Geometry: final body of the model. Coordinates: model frame, mm. A direction names the side the tool comes from. Give positions to 0.01 mm unless a question says otherwise; leave off trailing zeros. Loops run counter-clockwise (first coordinate to the right, second up) from the corner with the lowest first, then second, coordinate; pieces in that order, holes last. Notation, with made-up numbers: (73.25, 82.25) - (108.25, 82.25) arc R24 cw to (108.25, 106.25) - close; hole circle Ø5 at (-22.5, -37.75). An arc over 180 degrees is marked (long way). Answer in a Markdown table with one row per item.
from build123d import *

# Parameters (mm, degrees)
BOSS_EXTRUDE1_DEPTH = 36
SKETCH3_R           = 8.75
SKETCH3_R_2         = 8
CUT_EXTRUDE1_DEPTH  = 10
CUT_EXTRUDE2_DEPTH  = 2
SKETCH5_R           = 2.5
CUT_EXTRUDE3_DEPTH  = 1
SKETCH6_R           = 0.5
CUT_EXTRUDE4_DEPTH  = 5


with BuildPart() as part:
    # Sketch1 → Boss-Extrude1 (new body)
    with BuildSketch(Plane.XY):
        with BuildLine():
            Line((-77.5, 12.5), (77.5, 12.5))
            ThreePointArc((77.5, 12.5), (90, 0), (77.5, -12.5))
            Line((77.5, -12.5), (-77.5, -12.5))
            ThreePointArc((-77.5, -12.5), (-90, 0), (-77.5, 12.5))
        make_face()
    extrude(amount=-BOSS_EXTRUDE1_DEPTH)

    # Sketch3 → Cut-Extrude1 (cut)
    with BuildSketch(Plane.XY):
        with Locations((-28.5, 0)):
            Circle(SKETCH3_R)
        with Locations((18.5, 0)):
            Circle(SKETCH3_R_2)
        with Locations((44.5, 0)):
            Circle(SKETCH3_R_2)
    extrude(amount=-CUT_EXTRUDE1_DEPTH, mode=Mode.SUBTRACT)

    # Sketch4 → Cut-Extrude2 (cut)
    with BuildSketch(Plane.XY):
        with BuildLine():
            Line((-47.25, 9.5), (-20.75, 9.5))
            ThreePointArc((-20.75, 9.5), (-11.25, 0), (-20.75, -9.5))
            Line((-20.75, -9.5), (-47.25, -9.5))
            ThreePointArc((-47.25, -9.5), (-56.75, 0), (-47.25, 9.5))
        make_face()
        with BuildLine():
            Line((18, 9.5), (45, 9.5))
            ThreePointArc((45, 9.5), (54.5, 0), (45, -9.5))
            Line((45, -9.5), (18, -9.5))
            ThreePointArc((18, -9.5), (8.5, 0), (18, 9.5))
        make_face()
    extrude(amount=-CUT_EXTRUDE2_DEPTH, mode=Mode.SUBTRACT)

    # Sketch5 → Cut-Extrude3 (cut)
    with BuildSketch(Plane.XY):
        with Locations((72.5, -5.85958214)):
            Circle(SKETCH5_R)
        with Locations((-72.5, -5.85958214)):
            Circle(SKETCH5_R)
    extrude(amount=-CUT_EXTRUDE3_DEPTH, mode=Mode.SUBTRACT)

    # Sketch6 → Cut-Extrude4 (cut)
    with BuildSketch(Plane.XY):
        with Locations((-72.5, -5.85958214)):
            Circle(SKETCH6_R)
        with Locations((72.5, -5.85958214)):
            Circle(SKETCH6_R)
        with BuildLine():
            ThreePointArc((-71.394458403, -7.526248807), (-70.5, -5.85958214), (-71.394458403, -4.192915474))
            ThreePointArc((-71.394458403, -4.192915474), (-72.087510469, -4.333196741), (-71.947229202, -5.026248807))
            ThreePointArc((-71.947229202, -5.026248807), (-71.5, -5.85958214), (-71.947229202, -6.692915474))
            ThreePointArc((-71.947229202, -6.692915474), (-72.087510469, -7.385967539), (-71.394458403, -7.526248807))
        make_face()
        with BuildLine():
            ThreePointArc((-73.605541597, -4.192915474), (-74.5, -5.85958214), (-73.605541597, -7.526248807))
            ThreePointArc((-73.605541597, -7.526248807), (-72.912489531, -7.385967539), (-73.052770798, -6.692915474))
            ThreePointArc((-73.052770798, -6.692915474), (-73.5, -5.85958214), (-73.052770798, -5.026248807))
            ThreePointArc((-73.052770798, -5.026248807), (-72.912489531, -4.333196741), (-73.605541597, -4.192915474))
        make_face()
        with BuildLine():
            ThreePointArc((73.605541597, -7.526248807), (74.5, -5.85958214), (73.605541597, -4.192915474))
            ThreePointArc((73.605541597, -4.192915474), (72.912489531, -4.333196741), (73.052770798, -5.026248807))
            ThreePointArc((73.052770798, -5.026248807), (73.5, -5.85958214), (73.052770798, -6.692915474))
            ThreePointArc((73.052770798, -6.692915474), (72.912489531, -7.385967539), (73.605541597, -7.526248807))
        make_face()
        with BuildLine():
            ThreePointArc((71.394458403, -4.192915474), (70.5, -5.85958214), (71.394458403, -7.526248807))
            ThreePointArc((71.394458403, -7.526248807), (72.087510469, -7.385967539), (71.947229202, -6.692915474))
            ThreePointArc((71.947229202, -6.692915474), (71.5, -5.85958214), (71.947229202, -5.026248807))
            ThreePointArc((71.947229202, -5.026248807), (72.087510469, -4.333196741), (71.394458403, -4.192915474))
        make_face()
    extrude(amount=-CUT_EXTRUDE4_DEPTH, mode=Mode.SUBTRACT)


solid = part.part
Q1. Draft query along Y for faces 3 (the flat face through (1, -12.5, -18)), 4 (the cylindrical face through (-70.5, -5.9, -3)), 5 (the cylindrical face through (-90, 0, -18)). Return one class per face: pulls with the +Y half, pulls with the -Y half, needs draft (parallel to the pull), parting line crosses it, or undercut.
Check values:
| item | result |
|---|---|
| face 3 | pulls with the -Y half |
| face 4 | undercut |
| face 5 | parting line crosses it |
Q2. First-contact query: pin 1 (3 mm diameter, centred on x = 13, y = -5.5, fed in from +Z); pin 2 (0.8 mm diameter, centred on x = 72.5, y = -6, fed in from +Z); pin 3 (5 mm diameter, centred on x = -30.5, y = -1, fed in from +Z). Flat tips, straight axial feed; report the tip coordinate or a pass-through.
Check values:
| item | result |
|---|---|
| pin 1 | z = -2 |
| pin 2 | z = -1 |
| pin 3 | z = -10 |
Q3. Reachability of faces 1 (the flat face through (-1, 12.5, -18)), 2 (the flat face through (-39, 0, -2)) from +Z, -Z, +X, -X, +Y, -Y: full face, straight path, thin tool, end or side. Return the list, or none.
Check values:
| item | result |
|---|---|
| face 1 | +Z, -Z, +X, -X, +Y |
| face 2 | +Z |
Q4. Cut plane C-C (y = 6). Output: boundary loops of the cut face in (x, z), and give its area (3 significant figures).
Check values:
| item | result |
|---|---|
| outline | (-88.47, -36) - (88.47, -36) - (88.47, 0) - (52.37, 0) - (52.37, -2) - (49.79, -2) - (49.79, -10) - (39.21, -10) - (39.21, -2) - (23.79, -2) - (23.79, -10) - (13.21, -10) - (13.21, -2) - (10.63, -2) - (10.63, 0) - (-13.38, 0) - (-13.38, -2) - (-22.13, -2) - (-22.13, -10) - (-34.87, -10) - (-34.87, -2) - (-54.62, -2) - (-54.62, 0) - (-88.47, 0) - close |
| area | 5,930 mm² |
Q5. Cut plane B-B (x = -28.5). Output: boundary loops of the cut face in (y, z).
Check values:
| item | result |
|---|---|
| outline | (-12.5, -36) - (12.5, -36) - (12.5, 0) - (9.5, 0) - (9.5, -2) - (8.75, -2) - (8.75, -10) - (-8.75, -10) - (-8.75, -2) - (-9.5, -2) - (-9.5, 0) - (-12.5, 0) - close |
Q6. Cut plane A-A (z = -7). Output: boundary loops of the cut face in (x, y), and give its area (3 significant figures).
Check values:
| item | result |
|---|---|
| outline | (-77.5, -12.5) - (77.5, -12.5) arc R12.5 ccw to (77.5, 12.5) - (-77.5, 12.5) arc R12.5 ccw to start; hole circle Ø17.5 at (-28.5, 0); hole circle Ø16 at (18.5, 0); hole circle Ø16 at (44.5, 0) |
| area | 3,720 mm² |
Q7. Material intervals for line 1 along Y through (x, z) = (72.5, -0.4); line 2 along Y through (x, z) = (44, -3); line 3 along X through (y, z) = (-2.75, -4.5), sorted ascending.
Check values:
| item | result |
|---|---|
| line 1 | -12.5 to -8.36, -3.36 to 12.5 |
| line 2 | -12.5 to -7.98, 7.98 to 12.5 |
| line 3 | -89.69 to -36.81, -20.19 to 10.99, 26.01 to 36.99, 52.01 to 89.69 |
Q8. Cut plane D-D (z = -22). Output: boundary loops of the cut face in (x, y), and give its area (3 significant figures).
Check values:
| item | result |
|---|---|
| outline | (-77.5, -12.5) - (77.5, -12.5) arc R12.5 ccw to (77.5, 12.5) - (-77.5, 12.5) arc R12.5 ccw to start |
| area | 4,370 mm² |
